from build123d import *

# Parameters (mm, degrees)
SKETCH1_R           = 12.5
BOSS_EXTRUDE1_DEPTH = 2.5
SHELL1_T            = -1
SKETCH2_R           = 11.5
BOSS_EXTRUDE2_DEPTH = 0.5
SKETCH5_R           = 3.045955351
CUT_EXTRUDE3_DEPTH  = 10.5


with BuildPart() as part:
    # Sketch1 → Boss-Extrude1 (new body)
    with BuildSketch(Plane(origin=(0, 0, 0), x_dir=(1, 0, 0), z_dir=(0, 1, 0))):
        with Locations(Location((0, 0, 0), (0, 0, 270))):
            Circle(SKETCH1_R)
    extrude(amount=BOSS_EXTRUDE1_DEPTH)

    # Shell1
    shell1_openings = [part.faces().sort_by_distance(p)[0] for p in [
        (0, 0, 0),
    ]]
    offset(amount=SHELL1_T, openings=shell1_openings, kind=Kind.INTERSECTION)

    # Sketch2 → Boss-Extrude2 (add)
    with BuildSketch(Plane(origin=(0, 2.5, 0), x_dir=(1, 0, 0), z_dir=(0, 1, 0))):
        with Locations(Location((0, 0, 0), (0, 0, 270))):
            Circle(SKETCH2_R)
    extrude(amount=BOSS_EXTRUDE2_DEPTH)

    # Sketch4 → Revolve1 (revolve)
    with BuildSketch(Plane.XY, mode=Mode.PRIVATE) as revolve1_sk:
        Polygon((4.455880937, -1), (3.955880937, -1), (2.5, 3), (3, 3), align=None)
    revolve(revolve1_sk.sketch.rotate(Axis((0, 3, 0), (0, -1, 0)), 90), axis=Axis((0, 3, 0), (0, -1, 0)))

    # Sketch5 → Cut-Extrude3 (cut)
    with BuildSketch(Plane.XZ.offset(-1.5)):
        with Locations(Location((0, 0, 0), (0, 0, 270))):
            Circle(SKETCH5_R)
    extrude(amount=-CUT_EXTRUDE3_DEPTH, mode=Mode.SUBTRACT)


solid = part.part
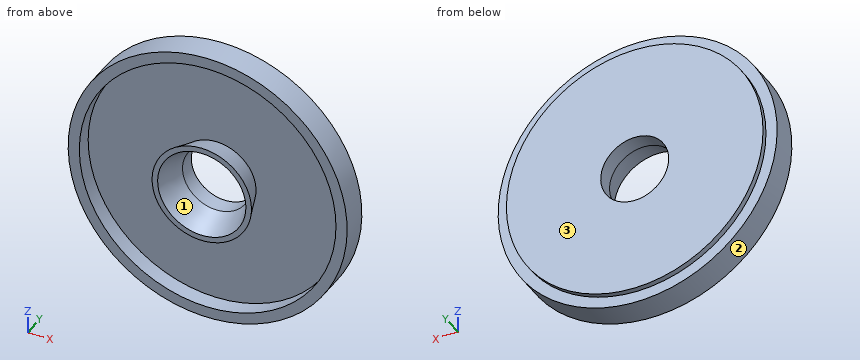
Could you check a few things on this model? Use its own coordinates, in mm. Face numbers are marked on the shaded views. Give positions to 0.01 mm unless a question says otherwise; leave off trailing zeros. Write each loop counter-clockwise with the first axis right and the second up, starting at its lowest first coordinate (ties: lowest second). Pieces come first, ordered by that corner, then holes. Notation, with made-up numbers: (79.25, 6) -> (131.25, 6) arc R14 cw to (131.25, 16) -> close; hole circle Ø7 at (28, 53). An arc over 180 degrees is marked (long way). Write each question's results on one line, items separated by ' | '. Start each with the question number.
Q1. We'd pull the mould along X, two halves only. Please class the marked faces 1, 2 and 3: +X half, -X half, draft (parallel to the pull), parting line (faces both ways), or undercut.
Q2. Suppose I cut it at D-D, the plane x = -10. List the corners of the cut face in (y, z) for me, and give its area (3 significant figures).
Q3. I need wall thicknesses on probe 1 along X at (y, z) = (1.9, 0); probe 2 along X at (y, z) = (0.5, 0); probe 3 along Z at (x, y) = (-1, 0.65). Which ranges of each line are inside material? Lowest first, please.
Q4. I'm going to push flat-ended pins straight in: pin 1 Ø1.5 at (x, y) = (-6.5, 2.5) entering from +Z; pin 2 Ø1 at (x, z) = (8, -3.5) entering from -Y; pin 3 Ø1.5 at (x, y) = (-2, 2) entering from +Z. Where does each tip first touch, or does it pass through?
Q5. Suppose I cut it at C-C, the plane z = 10.75. List the corners of the cut face in (x, y) for me.
Q6. Suppose I cut it at B-B, the plane z = 0. List the corners of the cut face in (x, y) for me.
Q7. Suppose I cut it at A-A, the plane x = 0. List the corners of the cut face in (y, z) for me.
Outcome:
1) face 1: undercut | face 2: parting line | face 3: draft
2) outline: (0, -7.5) -> (2.5, -7.5) -> (2.5, -5.68) -> (3, -5.68) -> (3, 5.68) -> (2.5, 5.68) -> (2.5, 7.5) -> (0, 7.5) -> (0, 5.68) -> (1.5, 5.68) -> (1.5, -5.68) -> (0, -5.68) -> close | area: 26.1 mm2
3) probe 1: -12.5 to -3.05, 3.05 to 12.5 | probe 2: -12.5 to -11.5, -3.91 to -3.41, 3.41 to 3.91, 11.5 to 12.5 | probe 3: -12.46 to -11.46, -3.72 to -3.2, 3.2 to 3.72, 11.46 to 12.46
4) pin 1: z = 11.1 | pin 2: y = 1.5 | pin 3: z = 12.44
5) outline: (-6.38, 0) -> (-4.09, 0) -> (-4.09, 1.5) -> (4.09, 1.5) -> (4.09, 0) -> (6.38, 0) -> (6.38, 2.5) -> (4.09, 2.5) -> (4.09, 3) -> (-4.09, 3) -> (-4.09, 2.5) -> (-6.38, 2.5) -> close
6) outline: (-12.5, 0) -> (-11.5, 0) -> (-11.5, 1.5) -> (-3.55, 1.5) -> (-4.46, -1) -> (-3.96, -1) -> (-3.05, 1.5) -> (-3.05, 3) -> (-11.5, 3) -> (-11.5, 2.5) -> (-12.5, 2.5) -> close; (3.05, 1.5) -> (3.96, -1) -> (4.46, -1) -> (3.55, 1.5) -> (11.5, 1.5) -> (11.5, 0) -> (12.5, 0) -> (12.5, 2.5) -> (11.5, 2.5) -> (11.5, 3) -> (3.05, 3) -> close
7) outline: (-1, -4.46) -> (1.5, -3.55) -> (1.5, -11.5) -> (0, -11.5) -> (0, -12.5) -> (2.5, -12.5) -> (2.5, -11.5) -> (3, -11.5) -> (3, -3.05) -> (1.5, -3.05) -> (-1, -3.96) -> close; (-1, 3.96) -> (1.5, 3.05) -> (3, 3.05) -> (3, 11.5) -> (2.5, 11.5) -> (2.5, 12.5) -> (0, 12.5) -> (0, 11.5) -> (1.5, 11.5) -> (1.5, 3.55) -> (-1, 4.46) -> close
